Can you work these out from the model? Positions are in its coordinate system, mm. A direction names the side the tool comes from. Coordinates: 2 decimals unless noted, no trailing zeros. Order: outer loops, then holes, each group sorted by start corner. A loop starts at its lowest first (then second) coordinate and runs counter-clockwise, first axis right, second up. Notation, with made-up numbers: (40.25, 63) -> (71.25, 63) arc R14 ccw to (71.25, 84) -> close; hole circle Ø11 at (78, -27). An arc over 180 degrees is marked (long way). Use a Markdown table: item, result. Add a question column.
1. Suppose I cut it at A-A, the plane x = 31.6. List the corners of the cut face in (y, z) for me.
2. Suppose I cut it at D-D, the plane x = 22. List the corners of the cut face in (y, z) for me.
3. We'd pull the mould along Y, two halves only. Please class faces 1 (the flat face through (19, -25, 0)), 2 (the cylindrical face through (0.079, -9.609, 43.274)), 3 (the flat face through (3.7, 0, 23.4)): pulls with the +Y half, pulls with the -Y half, needs draft (parallel to the pull), parting line crosses it, or undercut.
4. If I drill on line 1 along Y through (x, z) = (0.35, 40.3); line 2 along Z through (x, y) = (-0.65, -10); line 3 along Y through (x, z) = (14.45, 1.8), over which ranges is the centre line in solid material (lowest first)? Write a range as from..to.
5. For faces 4 (the flat face through (-1.4, -25, 46)), 5 (the flat face through (0, -25, 13)), 6 (the flat face through (22, -25, 6)), which set-ups out of +Z, -Z, +X, -X, +Y, -Y let a thin tool reach every point of the face, with its end or its side?
6. Suppose I cut it at C-C, the plane y = -30. List the corners of the cut face in (x, z) for me.
7. For pin 1 Ø5 at (y, z) = (-10, 40.3) entering from -X; pin 2 Ø2 at (y, z) = (-7.5, 16) entering from -X; pin 3 Ø3 at (x, y) = (8, -25.5) entering from +Z; pin 4 Ø9.5 at (x, y) = (14.45, -11.73) entering from +Z, each with a flat end and sliding along its axis, tell me the tip position at first contact or that it passes through.
8. Suppose I cut it at B-B, the plane z = 40.3. List the corners of the cut face in (x, y) for me.
```python
from build123d import *

# Parameters (mm, degrees)
F1_DEPTH       = 50
F3_D           = 6
F3_DEPTH       = 12
F3_CSINK_D     = 12
F3_CSINK_ANGLE = 90
F5_D           = 6
F5_DEPTH       = 12
F5_CSINK_D     = 12
F5_CSINK_ANGLE = 90
F6_SIZE        = 0.5
F7_SIZE        = 0.2


with BuildPart() as f1:
    # F0 (on Front) → F1 (new body)
    with BuildSketch(Plane.XZ):
        Polygon((0, 26), (0, 0), (38.6, 0), (38.6, 6), (4.6, 6), (4.6, 66), (-1.4, 66), (-1.4, 26), align=None)
    extrude(amount=F1_DEPTH)

    # F3
    with Locations(Plane.YZ.offset(4.6)):
        with Locations((-40, 40.3), (-10, 40.3)):
            CounterSinkHole(F3_D / 2, F3_CSINK_D / 2, depth=F3_DEPTH, counter_sink_angle=F3_CSINK_ANGLE)

    # F5
    with Locations(Plane.XY.offset(6)):
        with Locations((14.45, -11.727238), (31.6, -41.727238)):
            CounterSinkHole(F5_D / 2, F5_CSINK_D / 2, depth=F5_DEPTH, counter_sink_angle=F5_CSINK_ANGLE)

    # F6
    f6_edges = [f1.edges().sort_by_distance(p)[0] for p in [
        (4.6, -25, 66),
        (4.6, -50, 36),
        (4.6, 0, 36),
        (21.6, -50, 6),
        (38.6, -25, 6),
        (21.6, 0, 6),
    ]]
    chamfer(f6_edges, length=F6_SIZE)

    # F7
    f7_edges = [f1.edges().sort_by_distance(p)[0] for p in [
        (-1.4, -25, 26),
        (0, -25, 26),
    ]]
    chamfer(f7_edges, length=F7_SIZE)


solid = f1.part
```
Worked out:
| question | item | result |
|---|---|---|
| 1 | outline | (-50, 0) -> (-44.73, 0) -> (-44.73, 3) -> (-47.73, 6) -> (-49.5, 6) -> (-50, 5.5) -> close; (-38.73, 0) -> (0, 0) -> (0, 5.5) -> (-0.5, 6) -> (-35.73, 6) -> (-38.73, 3) -> close |
| 2 | outline | (-50, 0) -> (0, 0) -> (0, 5.5) -> (-0.5, 6) -> (-49.5, 6) -> (-50, 5.5) -> close |
| 3 | face 1 | needs draft |
| 3 | face 2 | undercut |
| 3 | face 3 | pulls with the +Y half |
| 4 | line 1 | y = -50..-43, -37..-13, -7..0 |
| 4 | line 2 | z = 26..37.3, 43.3..66 |
| 4 | line 3 | y = -50..-14.73, -8.73..0 |
| 5 | face 4 | +Z, -Z, -X, +Y, -Y |
| 5 | face 5 | -Z, -X, +Y, -Y |
| 5 | face 6 | +Z, +X, +Y, -Y |
| 6 | outline | (-1.4, 26.2) -> (-1.2, 26) -> (-0.2, 26) -> (0, 25.8) -> (0, 0) -> (38.6, 0) -> (38.6, 5.5) -> (38.1, 6) -> (4.6, 6) -> (4.6, 65.5) -> (4.1, 66) -> (-1.4, 66) -> close |
| 7 | pin 1 | passes through |
| 7 | pin 2 | stops at x = 0 |
| 7 | pin 3 | stops at z = 6 |
| 7 | pin 4 | stops at z = 4.75 |
| 8 | outline | (-1.4, -50) -> (4.1, -50) -> (4.6, -49.5) -> (4.6, -46) -> (1.6, -43) -> (-1.4, -43) -> close; (-1.4, -37) -> (1.6, -37) -> (4.6, -34) -> (4.6, -16) -> (1.6, -13) -> (-1.4, -13) -> close; (-1.4, -7) -> (1.6, -7) -> (4.6, -4) -> (4.6, -0.5) -> (4.1, 0) -> (-1.4, 0) -> close |
